Geometry check sheet. Reference: the model listing, model coordinates, mm. A direction names the side the tool comes from. Coordinates: 2 decimals unless noted, no trailing zeros. Write each loop counter-clockwise with the first axis right and the second up, starting at its lowest first coordinate (ties: lowest second). Pieces come first, ordered by that corner, then holes. Notation, with made-up numbers: M 50,34 L 70,34 A20 cw 70,58 Z; hole C 13.5,-29.5 d5. An arc over 180 degrees is marked long. Write item = value, one per line. Start each with the question number.
```python
from build123d import *

# Parameters (mm, degrees)
FILLET1_R             = 0.2
RECPAT_COUNT          = 2
RECPAT_ANGLE          = 90
CHAMFER_1_SIZE        = 0.5
CUT_EXTRUDE_START     = -1.932317225
CUT_EXTRUDE_1_DEPTH   = 0.992538955
CUT_EXTRUDE_1_2_DEPTH = 0.992538955
CUT_EXTRUDE_1_3_DEPTH = 0.992538955
CUT_EXTRUDE_1_4_DEPTH = 0.992538955


# Read off the part's stored shape, not the designer's step: Вытянуть1
with BuildPart() as part:
    # BodySke → Base-Revolve (revolve)
    with BuildSketch(Plane.XY, mode=Mode.PRIVATE) as base_revolve_sk:
        Polygon((3.05, 2), (3.05, 5), (2.05, 5), (2.05, 0), (28.05, 0), (28.05, 2), align=None)
    revolve(base_revolve_sk.sketch.rotate(Axis((-6.35, 0, 0), (1, 0, 0)), 90), axis=Axis((-6.35, 0, 0), (1, 0, 0)))

    # Fillet1
    fillet1_edges = [part.edges().sort_by_distance(p)[0] for p in [
        (3.05, 0, -2),
    ]]
    fillet(fillet1_edges, radius=FILLET1_R)

    # PanSke → Pan (revolve)
    with BuildSketch(Plane.XY):
        with BuildLine():
            Line((2.05, 4.424646879), (2.05, 0))
            Line((2.05, 0), (0, 0))
            ThreePointArc((0, 0), (0.537396082, 2.438237068), (2.05, 4.424646879))
        make_face()
    revolve(axis=Axis((0, 0, 0), (1, 0, 0)))

    # Sketch3 → Recess section 0
    with BuildSketch(Plane(origin=(0, 0, 0), x_dir=(0, 0, -1), z_dir=(1, 0, 0))):
        with BuildLine():
            Line((-0.515, 2.15), (0.515, 2.15))
            Line((0.515, 2.15), (0.515, -2.15))
            Line((0.515, -2.15), (-0.515, -2.15))
            Line((-0.515, -2.15), (-0.515, 2.15))
        make_face()
    # Sketch4 → Recess section 1
    with BuildSketch(Plane(origin=(2.34, 0, 0), x_dir=(0, 0, -1), z_dir=(1, 0, 0))):
        with BuildLine():
            Line((-0.37, 1.45), (0.37, 1.45))
            Line((0.37, 1.45), (0.37, -1.45))
            Line((0.37, -1.45), (-0.37, -1.45))
            Line((-0.37, -1.45), (-0.37, 1.45))
        make_face()
    recess = loft(mode=Mode.SUBTRACT)

    # RecPat: Recess ×2 about axis
    recpat_axis = Axis((0, 0, 0), (1, 0, 0))
    for i in range(1, RECPAT_COUNT):
        add(recess.rotate(recpat_axis, i * RECPAT_ANGLE / (RECPAT_COUNT - 1)), mode=Mode.SUBTRACT)

    # RecCorSke → RecessCore (revolve, cut)
    with BuildSketch(Plane.XY, mode=Mode.PRIVATE) as recesscore_sk:
        Polygon((0, 0), (0, 1.032809711), (2.6, 0.851), (2.876506661, 0), align=None)
    revolve(recesscore_sk.sketch.rotate(Axis((-3.175, 0, 0), (1, 0, 0)), 90), axis=Axis((-3.175, 0, 0), (1, 0, 0)), mode=Mode.SUBTRACT)

    # Фаска1
    chamfer_1_edges = [part.edges().sort_by_distance(p)[0] for p in [
        (28.05, 0, -2),
    ]]
    chamfer(chamfer_1_edges, length=CHAMFER_1_SIZE)

    # Вытянуть1 outline → Вытянуть1 (cut)
    with BuildSketch(Plane(origin=(0, 0, 0), x_dir=(0.9932989193126689, -0.08172287590474318, -0.08172287590474292), z_dir=(0.11557359946062105, 0.7023684015912586, 0.7023684015912564)).offset(CUT_EXTRUDE_START)):
        Polygon((-1, -0.919204654), (0.206895578, -0.216114133), (0.577867997, 0), (0.206895578, 0.216114133), (-1, 0.919204654), align=None)
    extrude(amount=CUT_EXTRUDE_1_DEPTH, mode=Mode.SUBTRACT)

    # Cut-Extrude 1 2 outline → Cut-Extrude 1 2 (cut)
    with BuildSketch(Plane(origin=(0, 0, 0), x_dir=(0.9932989193126689, -0.08172287590474318, 0.08172287590474292), z_dir=(0.11557359946062105, 0.7023684015912586, -0.7023684015912564)).offset(CUT_EXTRUDE_START)):
        Polygon((0.206895578, -0.216114133), (0.577867997, 0), (0.206895578, 0.216114133), (-1, 0.919204654), (-1, -0.919204654), align=None)
    extrude(amount=CUT_EXTRUDE_1_2_DEPTH, mode=Mode.SUBTRACT)

    # Cut-Extrude 1 3 outline → Cut-Extrude 1 3 (cut)
    with BuildSketch(Plane(origin=(0, 0, 0), x_dir=(0.9932989193126689, 0.08172287590474318, 0.08172287590474292), z_dir=(0.11557359946062105, -0.7023684015912586, -0.7023684015912564)).offset(CUT_EXTRUDE_START)):
        Polygon((0.206895578, -0.216114133), (0.577867997, 0), (0.206895578, 0.216114133), (-1, 0.919204654), (-1, -0.919204654), align=None)
    extrude(amount=CUT_EXTRUDE_1_3_DEPTH, mode=Mode.SUBTRACT)

    # Cut-Extrude 1 4 outline → Cut-Extrude 1 4 (cut)
    with BuildSketch(Plane(origin=(0, 0, 0), x_dir=(0.9932989193126689, 0.08172287590474318, -0.08172287590474292), z_dir=(0.11557359946062105, -0.7023684015912586, 0.7023684015912564)).offset(CUT_EXTRUDE_START)):
        Polygon((-1, -0.919204654), (0.206895578, -0.216114133), (0.577867997, 0), (0.206895578, 0.216114133), (-1, 0.919204654), align=None)
    extrude(amount=CUT_EXTRUDE_1_4_DEPTH, mode=Mode.SUBTRACT)


solid = part.part
```
Q1. Draft check along Y on faces 1 (the face through (2.543, -0.22, -4.995)), 2 (the face through (3.05, 1, -2.2)), 3 (the face through (2.863, -0.012, 0.039)). Enter one of: pulls with the +Y half, pulls with the -Y half, needs draft (parallel to the pull), parting line crosses it, or undercut.
Q2. Cross-section at C-C on y = 3. Enter the section's corners in (x, z), and give its area (3 significant figures).
Q3. Set-up check for faces 4 (the face through (15, 2, 0)), 5 (the face through (1.6, -0.6, -0.7)): record each of +Z, -Z, +X, -X, +Y, -Y from which the full face is reachable in a straight line by a thin tool's end or side.
Q4. Scan lines: L1, parallel to X at y = -2.75, z = -2.75; L2, parallel to X at y = 1, z = -2.25; L3, parallel to Z at x = 14, y = 0.5. Record each from-to range of solid material in increasing order.
Q5. Cross-section at B-B on x = 14.5. Enter the section's corners in (y, z).
Q6. Cross-section at A-A on z = 4. Enter the section's corners in (x, y), and give its area (3 significant figures).
Q7. Gauge pin test, flat ends, axial feed: pin 1 (2 mm diameter, centred on y = 1.5, z = 3.5, fed in from -X) (3 decimals); pin 2 (2 mm diameter, centred on y = 2.5, z = 1.5, fed in from +X); pin 3 (6 mm diameter, centred on x = 8.5, z = 1, fed in from -Y). Record the tip position at first contact, or that the pin passes through.
Values found:
q1.face_1 = parting line crosses it
q1.face_2 = needs draft
q1.face_3 = undercut
q2.outline = M 2.05,-4 L 3.05,-4 L 3.05,4 L 2.05,4 L 2.05,3.25 A4.96 ccw 2.05,-3.25 Z
q2.area = 13.4 mm²
q3.face_4 = +X
q3.face_5 = -X
q4.L1 = 1.5 to 3.05
q4.L2 = 0.55 to 3.05
q4.L3 = -1.94 to 1.94
q5.outline = C 0,0 d4
q6.outline = M 2.05,-3 L 3.05,-3 L 3.05,3 L 2.05,3 L 2.05,1.89 A4.2 ccw 2.05,-1.89 Z
q6.area = 7.15 mm²
q7.pin_1 = 0.725
q7.pin_2 = 27.63
q7.pin_3 = -2
